```python
from build123d import *

# Parameters (mm, degrees)
SKETCH2_W                 = 235
SKETCH2_H                 = 235
BOSS_EXTRUDE1_DEPTH       = 3
SKETCH3_W                 = 229
SKETCH3_H                 = 229
BOSS_EXTRUDE3_DEPTH       = 75
BOSS_EXTRUDE4_OUTLINE_W   = 229
BOSS_EXTRUDE4_OUTLINE_H   = 229
BOSS_EXTRUDE4_OUTLINE_R   = 1.5
BOSS_EXTRUDE4_OUTLINE_W_2 = 195
BOSS_EXTRUDE4_OUTLINE_H_2 = 195
BOSS_EXTRUDE4_DEPTH       = 3
CUT_EXTRUDE1_DEPTH        = 600
CUT_EXTRUDE1_DEPTH_BACK   = 600
SKETCH9_R                 = 11.255
SKETCH9_R_2               = 1.5
SKETCH12_W                = 235
SKETCH12_H                = 235
SKETCH12_W_2              = 195
SKETCH12_H_2              = 195
BOSS_EXTRUDE5_DEPTH       = 5


# Read off the part's stored shape, not the designer's step: Boss-Extrude4
with BuildPart() as part:
    # Sketch2 → Boss-Extrude1 (new body)
    with BuildSketch(Plane(origin=(0, 0, 0), x_dir=(1, 0, 0), z_dir=(0, 1, 0))):
        with Locations((117.5, -117.5)):
            Rectangle(SKETCH2_W, SKETCH2_H)
    extrude(amount=BOSS_EXTRUDE1_DEPTH)

    # Sketch3 → Boss-Extrude3 (add)
    with BuildSketch(Plane(origin=(0, 3, 0), x_dir=(1, 0, 0), z_dir=(0, 1, 0))):
        Polygon((3, 0), (0, 0), (0, -3), (0, -232), (0, -235), (3, -235), (232, -235), (235, -235), (235, -232), (235, -3), (235, 0), (232, 0), align=None)
        with Locations((117.5, -117.5)):
            Rectangle(SKETCH3_W, SKETCH3_H, mode=Mode.SUBTRACT)
    extrude(amount=BOSS_EXTRUDE3_DEPTH)

    # Sketch9 → Cut-Extrude1 (cut, two sides: drawn at the far end of the back side and taken through both)
    with BuildSketch(Plane(origin=(235, 0, 0), x_dir=(0, 0, -1), z_dir=(1, 0, 0)).offset(-CUT_EXTRUDE1_DEPTH_BACK)):
        with Locations((-195, 19)):
            Circle(SKETCH9_R)
        with Locations((-40, 19)):
            Circle(SKETCH9_R)
        with Locations((-185.341358162, 30.476525513)):
            Circle(SKETCH9_R_2)
        with Locations((-204.658641838, 7.523474487)):
            Circle(SKETCH9_R_2)
        with Locations((-49.658641838, 30.476525513)):
            Circle(SKETCH9_R_2)
        with Locations((-30.341358162, 7.523474487)):
            Circle(SKETCH9_R_2)
    extrude(amount=CUT_EXTRUDE1_DEPTH + CUT_EXTRUDE1_DEPTH_BACK, mode=Mode.SUBTRACT)



with BuildPart() as body_2:
    # Boss-Extrude4 outline → Boss-Extrude4 (new body)
    with BuildSketch(Plane(origin=(0, 78, 0), x_dir=(1, 0, 0), z_dir=(0, 1, 0))):
        with Locations((117.5, -117.5)):
            Rectangle(BOSS_EXTRUDE4_OUTLINE_W, BOSS_EXTRUDE4_OUTLINE_H)
        with Locations((53, -222)):
            Circle(BOSS_EXTRUDE4_OUTLINE_R, mode=Mode.SUBTRACT)
        with Locations((182, -222)):
            Circle(BOSS_EXTRUDE4_OUTLINE_R, mode=Mode.SUBTRACT)
        with Locations((53, -13)):
            Circle(BOSS_EXTRUDE4_OUTLINE_R, mode=Mode.SUBTRACT)
        with Locations((117.5, -117.5)):
            Rectangle(BOSS_EXTRUDE4_OUTLINE_W_2, BOSS_EXTRUDE4_OUTLINE_H_2, mode=Mode.SUBTRACT)
        with Locations((182, -13)):
            Circle(BOSS_EXTRUDE4_OUTLINE_R, mode=Mode.SUBTRACT)
    extrude(amount=BOSS_EXTRUDE4_DEPTH)


with BuildPart() as part_1:
    add(part.part)

    add(body_2.part)  # Boss-Extrude5 merges body 2
    # Sketch12 → Boss-Extrude5 (add)
    with BuildSketch(Plane.XZ.offset(-78)):
        with Locations((117.5, 117.5)):
            Rectangle(SKETCH12_W, SKETCH12_H)
        with Locations((117.5, 117.5)):
            Rectangle(SKETCH12_W_2, SKETCH12_H_2, mode=Mode.SUBTRACT)
    extrude(amount=BOSS_EXTRUDE5_DEPTH)


solid = part_1.part
```
Geometry: final body of the model. Coordinates: model frame, mm. A direction names the side the tool comes from. Round coordinates to 2 decimals unless told otherwise and drop trailing zeros. Loops run counter-clockwise (first coordinate to the right, second up) from the corner with the lowest first, then second, coordinate; pieces in that order, holes last. Notation, with made-up numbers: (43.25, -12) -> (95.25, -12) arc R21 ccw to (95.25, 3) -> close; hole circle Ø6 at (22, 21). An arc over 180 degrees is marked (long way). Use one line per item in the form item = value.
Item 1: Cut plane A-A on z = 40. Output: boundary loops of the cut face in (x, y) (3 decimals).
Evaluation:
outline = (0, 0) -> (235, 0) -> (235, 7.745) -> (232, 7.745) -> (232, 3) -> (3, 3) -> (3, 7.745) -> (0, 7.745) -> close; (0, 30.255) -> (3, 30.255) -> (3, 73) -> (20, 73) -> (20, 81) -> (3, 81) -> (3, 78) -> (0, 78) -> close; (215, 73) -> (232, 73) -> (232, 30.255) -> (235, 30.255) -> (235, 78) -> (232, 78) -> (232, 81) -> (215, 81) -> close
Item 2: Draft query along X for faces 1 (the flat face through (116, 3, 116)), 2 (the flat face through (119, 38, 0)), 3 (the flat face through (235, 38, 119)). Return one class per face: released by +X, released by -X, zero draft, split by the parting line, or undercut.
Evaluation:
face_1 = undercut
face_2 = zero draft
face_3 = released by +X
Item 3: Access query for faces 4 (the flat face through (116, 77, 20)), 5 (the cylindrical face through (233.479, 22.381, 29.265)), 6 (the flat face through (116, 38, 232)). Directions: +Z, -Z, +X, -X, +Y, -Y. A direction counts if a zero-diameter tool reaches every point of the face in a straight line with its end or side. Return the directions, or none.
Evaluation:
face_4 = +Y
face_5 = +X, -X
face_6 = none
Item 4: Contact query for flat-ended pins moving along their axis: pin 1 Ø5 at (x, z) = (27.5, 112.5) entering from +Y; pin 2 Ø5 at (y, z) = (30.48, 49.66) entering from -X; pin 3 Ø2.5 at (x, z) = (182, 13) entering from +Y; pin 4 Ø3.5 at (y, z) = (80, 83.5) entering from +X. Output: stop coordinate, or through.
Evaluation:
pin_1 = 3
pin_2 = 0
pin_3 = 78
pin_4 = 232
Item 5: Cut plane C-C on x = 81.5. Output: boundary loops of the cut face in (y, z).
Evaluation:
outline = (0, 0) -> (78, 0) -> (78, 3) -> (81, 3) -> (81, 20) -> (73, 20) -> (73, 3) -> (3, 3) -> (3, 232) -> (73, 232) -> (73, 215) -> (81, 215) -> (81, 232) -> (78, 232) -> (78, 235) -> (0, 235) -> close
Item 6: Material intervals for probe 1 along Z at (x, y) = (182, 80.4); probe 2 along X at (y, z) = (80.1, 222); probe 3 along Z at (x, y) = (193.5, 68), sorted ascending.
Evaluation:
probe_1 = 3 to 11.5, 14.5 to 20, 215 to 220.5, 223.5 to 232
probe_2 = 3 to 51.5, 54.5 to 180.5, 183.5 to 232
probe_3 = 0 to 3, 232 to 235
Item 7: Cut plane B-B on y = 19. Output: boundary loops of the cut face in (x, z) (3 decimals).
Evaluation:
outline = (0, 0) -> (235, 0) -> (235, 28.745) -> (232, 28.745) -> (232, 3) -> (3, 3) -> (3, 28.745) -> (0, 28.745) -> close; (0, 51.255) -> (3, 51.255) -> (3, 183.745) -> (0, 183.745) -> close; (0, 206.255) -> (3, 206.255) -> (3, 232) -> (232, 232) -> (232, 206.255) -> (235, 206.255) -> (235, 235) -> (0, 235) -> close; (232, 51.255) -> (235, 51.255) -> (235, 183.745) -> (232, 183.745) -> close
Item 8: Cut plane D-D on y = 54. Output: boundary loops of the cut face in (x, z).
Evaluation:
outline = (0, 0) -> (235, 0) -> (235, 235) -> (0, 235) -> close; hole (3, 3) -> (232, 3) -> (232, 232) -> (3, 232) -> close
